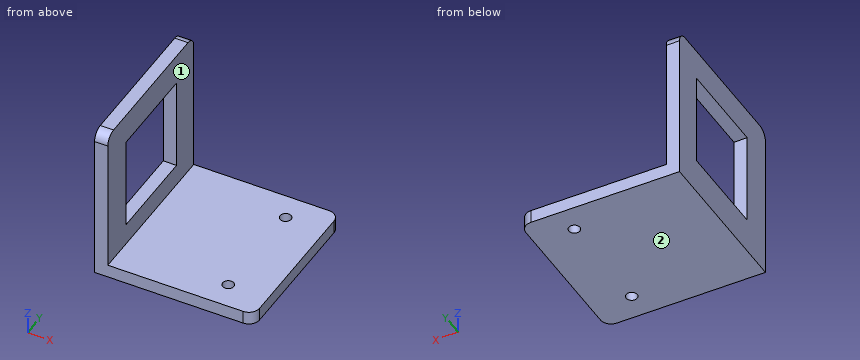
```python
from build123d import *

# Parameters (mm, degrees)
F1_DEPTH = 76.2
F2_W     = 44.8056
F2_H     = 44.8056
F3_DEPTH = 25.4
F5_D     = 5.334
F5_DEPTH = 12.7
F6_R     = 5.08


with BuildPart() as f1:
    # F0 (on Front) → F1 (new body)
    with BuildSketch(Plane.XZ):
        Polygon((0, 76.2), (0, 0), (76.2, 0), (76.2, 6.35), (6.35, 6.35), (6.35, 76.2), align=None)
    extrude(amount=F1_DEPTH)

    # F2 (on face) → F3 (cut)
    with BuildSketch(Plane(origin=(0, 0, 0), x_dir=(0, -1, 0), z_dir=(-1, 0, 0))):
        with Locations((37.6428, 39.1922)):
            Rectangle(F2_W, F2_H)
    extrude(amount=-F3_DEPTH, mode=Mode.SUBTRACT)

    # F5
    with Locations(Plane.XY.offset(6.35)):
        with Locations((57.15, -12.7), (57.15, -63.5)):
            Hole(F5_D / 2, depth=F5_DEPTH)

    # F6
    f6_edges = [f1.edges().sort_by_distance(p)[0] for p in [
        (3.175, 0, 76.2),
        (3.175, -76.2, 76.2),
        (76.2, -76.2, 3.175),
        (76.2, 0, 3.175),
    ]]
    fillet(f6_edges, radius=F6_R)


solid = f1.part
```
Part model, mm, in its own coordinate system. Face numbers are marked on the shaded views. A direction names the side the tool comes from. Round coordinates to 2 decimals unless told otherwise and drop trailing zeros. Write each loop counter-clockwise with the first axis right and the second up, starting at its lowest first coordinate (ties: lowest second). Pieces come first, ordered by that corner, then holes.
Item 1: Cut at C-C, the plane y = -63.5. Give the cut face in (x, z), plus the area to 3 significant figures.
Results:
outline: (0, 0) - (54.48, 0) - (54.48, 6.35) - (6.35, 6.35) - (6.35, 76.2) - (0, 76.2) - close; (59.82, 0) - (76.2, 0) - (76.2, 6.35) - (59.82, 6.35) - close
area: 894 mm2
Item 2: Cut at B-B, the plane z = 19. Give the cut face in (x, y).
Results:
outline: (0, -76.2) - (6.35, -76.2) - (6.35, -60.05) - (0, -60.05) - close; (0, -15.24) - (6.35, -15.24) - (6.35, 0) - (0, 0) - close
Item 3: Probe L1, parallel to Y at x = 57, z = 2; L2, parallel to Z at x = 9.5, y = -34.5; L3, parallel to X at y = -63, z = 4. List the from-to ranges inside material, lowest first.
Results:
L1: y = -76.2 to -66.16, -60.84 to -15.36, -10.04 to 0
L2: z = 0 to 6.35
L3: x = 0 to 54.53, 59.77 to 76.2
Item 4: Cut at A-A, the plane y = -50. Give the cut face in (x, z) (3 decimals), plus the area to 3 significant figures.
Results:
outline: (0, 0) - (76.2, 0) - (76.2, 6.35) - (6.35, 6.35) - (6.35, 16.789) - (0, 16.789) - close; (0, 61.595) - (6.35, 61.595) - (6.35, 76.2) - (0, 76.2) - close
area: 643 mm2
Item 5: Cut at D-D, the plane x = 43.5. Give the cut face in (y, z).
Results:
outline: (-76.2, 0) - (0, 0) - (0, 6.35) - (-76.2, 6.35) - close
Item 6: Drop flat-ended pins along their axis: pin 1 Ø8 at (y, z) = (-29.5, 13.5) entering from -X; pin 2 Ø5 at (x, y) = (29.5, -65.5) entering from +Z. Give the stop position or say it passes through.
Results:
pin 1: stops at x = 0
pin 2: stops at z = 6.35
Item 7: Which spindle directions (+Z, -Z, +X, -X, +Y, -Y) get a long thin tool onto all of the face, cutting with end or side? Do the marked faces 1 and 2. Say none if no direction does.
Results:
face 1: +Z, +X, +Y, -Y
face 2: -Z, +X, -X, +Y, -Y
